Autodesk Inventor part; units mm, degrees
ref_plane "YZ Plane" through (0, 0, 0) normal (1, 0, 0) x (0, 1, 0)
ref_plane "XZ Plane" through (0, 0, 0) normal (0, 1, 0) x (-1, 0, 0)
ref_plane "XY Plane" through (0, 0, 0) normal (0, 0, 1) x (1, 0, 0)
sketch "Esboço1" plane through (0, 0, 0) normal (0, 0, 1) x (1, 0, 0)
  circle A0 centre (0, 0) radius 27.5
  dimension "d0" = 55
extrude "Extrusão1" add sketch "Esboço1" along normal blind 45
sketch "Esboço2" plane through (0, 0, 45) normal (0, 0, 1) x (1, 0, 0)
  circle A0 centre (0, 0) radius 45
  dimension "d3" = 90
extrude "Extrusão2" add sketch "Esboço2" along normal blind 12
sketch "Esboço3" plane through (0, 0, 57) normal (0, 0, 1) x (1, 0, 0)
  circle A0 centre (35, 0) radius 4.5
  circle A1 centre (0, 35) radius 4.5
  circle A2 centre (-35, 0) radius 4.5
  circle A3 centre (0, -35) radius 4.5
  point P0 (0, 0)
  dimension "d7" = 9
  dimension "d8" = 35
  dimension "d11" = 360
extrude "Extrusão3" cut sketch "Esboço3" against normal blind 17.5
sketch "Esboço4" plane through (0, 0, 57) normal (0, 0, 1) x (1, 0, 0)
  circle A0 centre (0, 0) radius 27.5
  circle A1 centre (0, 0) radius 20
  dimension "d15" = 40
extrude "Extrusão4" add sketch "Esboço4" along normal blind 8 contours A1
sketch "Esboço6" plane through (0, 0, 0) normal (0, 0, -1) x (-1, 0, 0)
  line L0 (0, 10) -> (0, -10) construction
  line L1 (7.76, 10) -> (7.76, -10)
  line L2 (-7.76, -10) -> (-7.76, 10)
  arc A0 (7.76, 10) -> (-7.76, 10) centre (0, 10) ccw
  arc A1 (-7.76, -10) -> (7.76, -10) centre (0, -10) ccw
  point P0 (0, 0)
  point P1 (0, 0)
  dimension "d24" = 7.76
  dimension "d25" = 20
  dimension "d26" = 0
  dimension "d27" = 0
extrude "Extrusão5" cut sketch "Esboço6" against normal blind 10 draft -10
properties part number "Matriz inferior do Ferramental"
Can you work these out from the model? Positions are in its coordinate system, mm. A direction names the side the tool comes from. Give positions to 0.01 mm unless a question says otherwise; leave off trailing zeros. Order: outer loops, then holes, each group sorted by start corner. A loop starts at its lowest first (then second) coordinate and runs counter-clockwise, first axis right, second up. Notation, with made-up numbers: (8, 88.5) - (46, 88.5) arc R26 cw to (46, 115.5) - close; hole circle Ø8 at (85, 24.25). An arc over 180 degrees is marked (long way). Use a Markdown table: item, result. Add a question column.
Q1. On a 3-axis mill with a long thin cutter (end or side, diameter ignored), from which of +Z, -Z, +X, -X, +Y, -Y can I reach the whole of each face in a straight line? I mean faces 1 (the cylindrical face through (-5.961, 26.846, 22.185)), 2 (the flat face through (-21, 1, 57)), 3 (the cylindrical face through (39.292, 1.352, 51.084)). Say none if no direction works.
Q2. If we section it at B-B on y = 0: Write out the boundary of the cut face in (x, z).
Q3. I'm going to push flat-ended pins straight in: pin 1 (12 mm diameter, centred on x = 21.5, z = 40.5, fed in from +Y); pin 2 (10.5 mm diameter, centred on x = -35, y = 0, fed in from +Z); pin 3 (5 mm diameter, centred on x = 24, z = 48, fed in from -Y); pin 4 (8 mm diameter, centred on x = 0, y = -35, fed in from +Z). Where does each tip first touch, or does it pass through?
Q4. Please list where these lines run through material, in increasing order: line 1 along Y through (x, z) = (0, 52); line 2 along Z through (x, y) = (-31, 31); line 3 along X through (y, z) = (-16, 4.5).
Q5. If we section it at C-C on x = -35: Write out the boundary of the cut face in (y, z).
Q6. If we mould it in two halves opening along X, with no side actions, what happens to faces 4 (the cylindrical face through (-4.336, 19.524, 60.944)), 5 (the flat face through (-21, -19, 45)), 6 (the flat face through (-6.89, 0.14, 4.93))? For each: released by +X, released by -X, zero draft, split by the parting line, or undercut.
Q7. If we section it at A-A on x = 0: Write out the boundary of the cut face in (y, z), plus the area to 3 significant figures.
Answers follow:
| question | item | result |
|---|---|---|
| 1 | face 1 | -Z |
| 1 | face 2 | +Z |
| 1 | face 3 | +Z, -Z |
| 2 | outline | (-45, 45) - (-39.5, 45) - (-39.5, 57) - (-45, 57) - close; (-30.5, 45) - (-27.5, 45) - (-27.5, 0) - (-7.76, 0) - (-6, 10) - (6, 10) - (7.76, 0) - (27.5, 0) - (27.5, 45) - (30.5, 45) - (30.5, 57) - (20, 57) - (20, 65) - (-20, 65) - (-20, 57) - (-30.5, 57) - close; (39.5, 45) - (45, 45) - (45, 57) - (39.5, 57) - close |
| 3 | pin 1 | stops at y = 41.44 |
| 3 | pin 2 | stops at z = 57 |
| 3 | pin 3 | stops at y = -39.53 |
| 3 | pin 4 | passes through |
| 4 | line 1 | y = -45 to -39.5, -30.5 to 30.5, 39.5 to 45 |
| 4 | line 2 | z = 45 to 57 |
| 4 | line 3 | x = -22.37 to -3.54, 3.54 to 22.37 |
| 5 | outline | (-28.28, 45) - (-4.5, 45) - (-4.5, 57) - (-28.28, 57) - close; (4.5, 45) - (28.28, 45) - (28.28, 57) - (4.5, 57) - close |
| 6 | face 4 | split by the parting line |
| 6 | face 5 | zero draft |
| 6 | face 6 | undercut |
| 7 | outline | (-45, 45) - (-39.5, 45) - (-39.5, 57) - (-45, 57) - close; (-30.5, 45) - (-27.5, 45) - (-27.5, 0) - (-17.76, 0) - (-16, 10) - (16, 10) - (17.76, 0) - (27.5, 0) - (27.5, 45) - (30.5, 45) - (30.5, 57) - (20, 57) - (20, 65) - (-20, 65) - (-20, 57) - (-30.5, 57) - close; (39.5, 45) - (45, 45) - (45, 57) - (39.5, 57) - close |
| 7 | area | 3,320 mm^2 |
